Build history of the part. All positions in model axes, mm. Face numbers are marked on the shaded views. A direction names the side the tool comes from. Give positions to 0.01 mm unless a question says otherwise; leave off trailing zeros. Loops run counter-clockwise (first coordinate to the right, second up) from the corner with the lowest first, then second, coordinate; pieces in that order, holes last.
1) Flat gauge pin, fed straight in: P1, Ø3, axis at x = 14.5, y = -1, coming from the +Z side. Where does the tip first touch, or does it go through?
2) 3-axis set-ups, long thin cutter, end or side, ignore diameter. For the marked faces 1 and 2: which of +Z, -Z, +X, -X, +Y, -Y reach the whole face in a straight line?
3) Band-saw the part on C-C on y = -2.25. List the corners of the cut face in (x, z) (3 decimals).
4) Wall check: line 1 (Y direction, x = 16, z = 1.25); line 2 (Z direction, x = 2, y = 1.75) (3 decimals); line 3 (Z direction, x = 24, y = 2) (3 decimals). Give the ranges that are in metal, low to high.
5) Band-saw the part on A-A on z = 0.75. List the corners of the cut face in (x, y), then the cut area to 3 significant figures.
6) Two-plate mould, pull along Z, no slides. Class the marked faces 3, 4, 5 and 6: +Z half, -Z half, draft (parallel to the pull), parting line (faces both ways), or undercut.
7) Band-saw the part on D-D on z = 3.75. List the corners of the cut face in (x, y).
8) Band-saw the part on B-B on x = 24. List the corners of the cut face in (y, z) (3 decimals), then the cut area to 3 significant figures.
```python
from build123d import *

# Parameters (mm, degrees)
SKETCH1_W           = 3.81
SKETCH1_H           = 5.588
BOSS_EXTRUDE1_DEPTH = 33.02


with BuildPart() as part:
    # Sketch1 → Boss-Extrude1 (new body)
    with BuildSketch(Plane(origin=(0, 0, 0), x_dir=(0, 0, -1), z_dir=(1, 0, 0))):
        Polygon((-2.742413779, 4.75), (-5.484827557, 0), (-2.742413779, -4.75), (2.742413779, -4.75), (5.484827557, 0), (2.742413779, 4.75), align=None)
        Rectangle(SKETCH1_W, SKETCH1_H, mode=Mode.SUBTRACT)
    extrude(amount=BOSS_EXTRUDE1_DEPTH)


solid = part.part
```
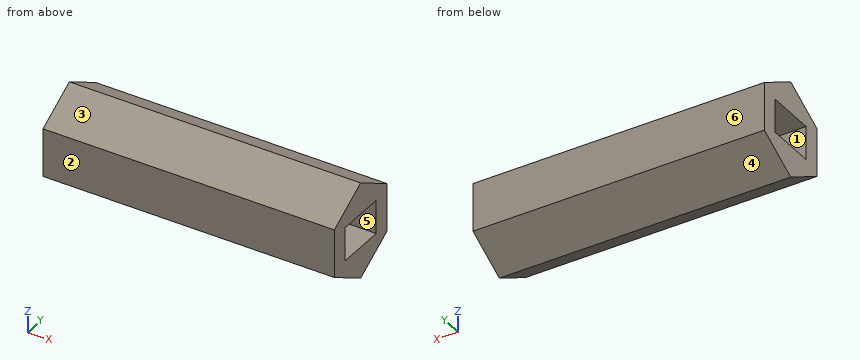
Findings below:
1. P1: stops at z = 5.48
2. face 1: +X, -X
2. face 2: +Z, -Z, +X, -X, -Y
3. outline: (0, -4.186) - (33.02, -4.186) - (33.02, -1.905) - (0, -1.905) - close; (0, 1.905) - (33.02, 1.905) - (33.02, 4.186) - (0, 4.186) - close
4. line 1: y = -4.75 to -2.79, 2.79 to 4.75
4. line 2: z = -4.474 to -1.905, 1.905 to 4.474
4. line 3: z = -4.33 to -1.905, 1.905 to 4.33
5. outline: (0, -4.75) - (33.02, -4.75) - (33.02, -2.79) - (0, -2.79) - close; (0, 2.79) - (33.02, 2.79) - (33.02, 4.75) - (0, 4.75) - close
5. area: 129 mm2
6. face 3: +Z half
6. face 4: -Z half
6. face 5: undercut
6. face 6: draft
7. outline: (0, -3) - (33.02, -3) - (33.02, 3) - (0, 3) - close
8. outline: (-4.75, -2.742) - (0, -5.485) - (4.75, -2.742) - (4.75, 2.742) - (0, 5.485) - (-4.75, 2.742) - close; hole (-2.794, -1.905) - (2.794, -1.905) - (2.794, 1.905) - (-2.794, 1.905) - close
8. area: 56.9 mm2
